```python
from build123d import *

# Parameters (mm, degrees)
EXTRUDE_1_DEPTH             = 15
HOLE_WIZARD_M81_D           = 9
HOLE_WIZARD_M81_CBORE_D     = 15
HOLE_WIZARD_M81_CBORE_DEPTH = 8.6
CHAMFER_1_SIZE              = 10


with BuildPart() as part:
    # Эскиз1 → Бобышка-Вытянуть1 (new, symmetric)
    with BuildSketch(Plane.XY):
        with BuildLine():
            Line((-15, 20), (-55, 20))
            Line((-55, 20), (-55, 40))
            Line((-55, 40), (55, 40))
            Line((55, 40), (55, 20))
            Line((55, 20), (15, 20))
            ThreePointArc((15, 20), (0, 25), (-15, 20))
        make_face()
    extrude(amount=EXTRUDE_1_DEPTH, both=True)

    # Цековка для винта с внутренним шестигранником M81 (through all)
    with Locations(Plane(origin=(0, 40, 0), x_dir=(1, 0, 0), z_dir=(0, 1, 0))):
        with Locations((0, 0), (-30, 0), (30, 0)):
            CounterBoreHole(HOLE_WIZARD_M81_D / 2, HOLE_WIZARD_M81_CBORE_D / 2, HOLE_WIZARD_M81_CBORE_DEPTH)

    # Фаска1
    chamfer_1_edges = [part.edges().sort_by_distance(p)[0] for p in [
        (-55, 40, 0),
        (55, 40, 0),
    ]]
    chamfer(chamfer_1_edges, length=CHAMFER_1_SIZE)


solid = part.part
```
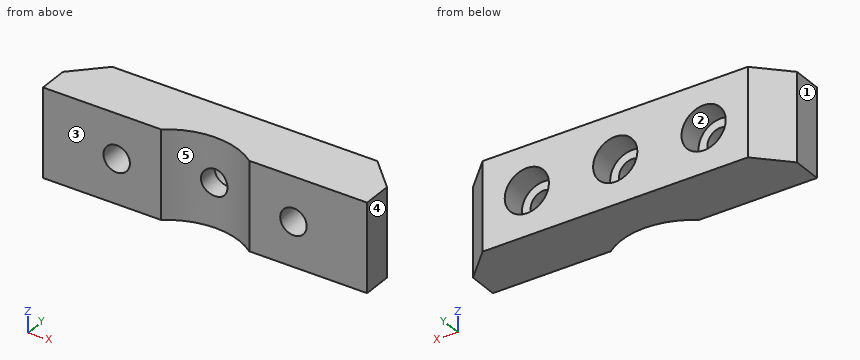
Model file for the job. Use its own axes, mm. Face numbers are marked on the shaded views. A direction names the side the tool comes from. Give positions to 0.01 mm unless a question says otherwise; leave off trailing zeros. Order: outer loops, then holes, each group sorted by start corner. A loop starts at its lowest first (then second) coordinate and runs counter-clockwise, first axis right, second up.
1) Pin check, flat tips, straight feed: pin 1 (11.5 mm diameter, centred on x = 30, z = 0, fed in from +Y); pin 2 (5 mm diameter, centred on x = -4, z = -3.5, fed in from -Y); pin 3 (2 mm diameter, centred on y = 31.5, z = 7.5, fed in from +X). Stop position of each tip, or through.
2) Saw through at D-D, the plane z = -9.5. Write the cut outline in (x, y), then the cut area to 3 significant figures.
3) Mould opens along X. For the marked faces 3, 4 and 5 say: +X half, -X half, draft (parallel to the pull), parting line (faces both ways), or undercut.
4) Wall check: probe 1 along X at (y, z) = (22.25, -3); probe 2 along X at (y, z) = (28.25, -4); probe 3 along Z at (x, y) = (-30, 33.75). Give the ranges that are in metal, low to high.
5) Saw through at A-A, the plane y = 28. Write the cut outline in (x, z), then the cut area to 3 significant figures.
6) Saw through at C-C, the plane z = 0. Count the separate pieces of the cut face and the enclosed holes in it, then the cut area to 3 significant figures.
7) Saw through at B-B, the plane x = -30. Write the cut outline in (y, z), then the cut area to 3 significant figures.
8) 3-axis set-ups, long thin cutter, end or side, ignore diameter. For the marked faces 1 and 2: which of +Z, -Z, +X, -X, +Y, -Y reach the whole face in a straight line?
Computed:
1. pin 1: stops at y = 31.4
1. pin 2: stops at y = 24.14
1. pin 3: stops at x = 54.5
2. outline: (-55, 20) - (-15, 20) arc R25 cw to (15, 20) - (55, 20) - (55, 30) - (45, 40) - (-45, 40) - (-55, 30) - close
2. area: 2,000 mm2
3. face 3: draft
3. face 4: +X half
3. face 5: undercut
4. probe 1: x = -55 to -33.35, -26.65 to -11.4, 11.4 to 26.65, 33.35 to 55
4. probe 2: x = -55 to -32.06, -27.94 to -2.06, 2.06 to 27.94, 32.06 to 55
4. probe 3: z = -15 to -7.5, 7.5 to 15
5. outline: (-55, -15) - (55, -15) - (55, 15) - (-55, 15) - close; hole circle Ø9 at (-30, 0); hole circle Ø9 at (0, 0); hole circle Ø9 at (30, 0)
5. area: 3,110 mm2
6. separate pieces: 4
6. enclosed holes: 0
6. area: 1,350 mm2
7. outline: (20, -15) - (40, -15) - (40, -7.5) - (31.4, -7.5) - (31.4, -4.5) - (20, -4.5) - close; (20, 4.5) - (31.4, 4.5) - (31.4, 7.5) - (40, 7.5) - (40, 15) - (20, 15) - close
7. area: 368 mm2
8. face 1: +Z, -Z, -X, +Y, -Y
8. face 2: +Y
